Read the model definition and answer for the solid it produces. Units are mm, in the model's axes. A direction names the side the tool comes from. Give positions to 0.01 mm unless a question says otherwise; leave off trailing zeros. Write each loop counter-clockwise with the first axis right and the second up, starting at its lowest first coordinate (ties: lowest second). Pieces come first, ordered by that corner, then holes. Notation, with made-up numbers: M 60,89.25 L 107,89.25 A18 ccw 107,113.25 Z; hole C 74,15.5 d8. An arc over 180 degrees is marked long. Answer as CSV lines item,"result". Start each with the question number.
```python
from build123d import *

# Parameters (mm, degrees)
PROFILE_W                = 12.7
PROFILE_H                = 22.86
PROFILE_W_2              = 6.35
PROFILE_H_2              = 12.7
BOSS_EXTRUDE1_DEPTH      = 12.7
SKETCH7_W                = 19.05
SKETCH7_H                = 12.7
BOSS_EXTRUDE2_DEPTH      = 25.4
CUT_EXTRUDE1_DEPTH       = 37.45585824
CUT_EXTRUDE1_DEPTH_BACK  = 37.45585824
SCREWHOLE_R              = 2.159
CUT_EXTRUDE2_START       = -4.064
SKETCH3_R                = 3.683
SKETCH3_R_2              = 2.159
CUT_EXTRUDE2_DEPTH       = 4.064
BOSS_EXTRUDE4_DEPTH      = 31.75
BOSS_EXTRUDE4_DEPTH_BACK = 31.75
SKETCH11_W               = 12.7
SKETCH11_H               = 22.86
SKETCH14_R               = 2.7051
CUT_EXTRUDE3_DEPTH       = 8.89
SKETCH13_R               = 1.143
CUT_EXTRUDE4_DEPTH       = 8.89
FILLET1_R                = 6.35


with BuildPart() as part:
    # Profile → Boss-Extrude1 (new, symmetric)
    with BuildSketch(Plane.XY):
        with Locations((0, 11.43)):
            Rectangle(PROFILE_W, PROFILE_H)
        with Locations((3.175, -6.35)):
            Rectangle(PROFILE_W_2, PROFILE_H_2)
    extrude(amount=BOSS_EXTRUDE1_DEPTH, both=True)

    # Sketch7 → Boss-Extrude2 (add)
    with BuildSketch(Plane.XY.offset(12.7)):
        with Locations((-9.525, -6.35)):
            Rectangle(SKETCH7_W, SKETCH7_H)
    extrude(amount=-BOSS_EXTRUDE2_DEPTH)

    # ScrewHole → Cut-Extrude1 (cut, two sides: drawn at the far end of the back side and taken through both)
    with BuildSketch(Plane.ZY.offset(19.05).offset(-CUT_EXTRUDE1_DEPTH_BACK)):
        with Locations(Location((6.35, -6.477, 0), (0, 0, 270))):
            Circle(SCREWHOLE_R)
        with Locations(Location((-6.35, -6.477, 0), (0, 0, 270))):
            Circle(SCREWHOLE_R)
    extrude(amount=CUT_EXTRUDE1_DEPTH + CUT_EXTRUDE1_DEPTH_BACK, mode=Mode.SUBTRACT)

    # Sketch3 → Cut-Extrude2 (cut)
    # profile 1 of 2: a face of its own
    with BuildSketch(Plane(origin=(6.35, 0, 0), x_dir=(0, 0, -1), z_dir=(1, 0, 0)).offset(CUT_EXTRUDE2_START)):
        with Locations(Location((-6.35, -6.477, 0), (0, 0, 90))):
            Circle(SKETCH3_R)
        with Locations(Location((-6.35, -6.477, 0), (0, 0, 270))):
            Circle(SKETCH3_R_2, mode=Mode.SUBTRACT)
    # profile 2 of 2: a face of its own
    with BuildSketch(Plane(origin=(6.35, 0, 0), x_dir=(0, 0, -1), z_dir=(1, 0, 0)).offset(CUT_EXTRUDE2_START)):
        with Locations(Location((6.35, -6.477, 0), (0, 0, 90))):
            Circle(SKETCH3_R)
    extrude(amount=CUT_EXTRUDE2_DEPTH, mode=Mode.SUBTRACT)

    # Sketch11 → Boss-Extrude4 (add, two sides: drawn at the far end of the back side and taken through both)
    with BuildSketch(Plane.XY.offset(-BOSS_EXTRUDE4_DEPTH_BACK)):
        with Locations((0, 11.43)):
            Rectangle(SKETCH11_W, SKETCH11_H)
    extrude(amount=BOSS_EXTRUDE4_DEPTH + BOSS_EXTRUDE4_DEPTH_BACK)

    # Sketch14 → Cut-Extrude3 (cut)
    with BuildSketch(Plane(origin=(6.35, 0, 0), x_dir=(0, 0, -1), z_dir=(1, 0, 0))):
        with Locations(Location((-25.4, 11.43, 0), (0, 0, 90))):
            Circle(SKETCH14_R)
        with Locations(Location((0, 11.43, 0), (0, 0, 90))):
            Circle(SKETCH14_R)
    extrude(amount=-CUT_EXTRUDE3_DEPTH, mode=Mode.SUBTRACT)

    # Sketch13 → Cut-Extrude4 (cut)
    with BuildSketch(Plane.ZY.offset(6.35)):
        with Locations(Location((-26.67, 17.78, 0), (0, 0, 270))):
            Circle(SKETCH13_R)
        with Locations(Location((-6.35, 17.78, 0), (0, 0, 270))):
            Circle(SKETCH13_R)
        with Locations(Location((-6.35, 5.08, 0), (0, 0, 270))):
            Circle(SKETCH13_R)
        with Locations(Location((-26.67, 5.08, 0), (0, 0, 270))):
            Circle(SKETCH13_R)
    extrude(amount=-CUT_EXTRUDE4_DEPTH, mode=Mode.SUBTRACT)

    # Fillet1
    fillet1_edges = [part.edges().sort_by_distance(p)[0] for p in [
        (-6.35, -12.7, -12.7),
        (-6.35, -12.7, 12.7),
        (0, 0, 31.75),
        (0, 22.86, 31.75),
        (0, 22.86, -31.75),
        (0, 0, -31.75),
        (0, 0, -12.7),
        (0, 0, 12.7),
    ]]
    fillet(fillet1_edges, radius=FILLET1_R - 0.0001)  # a hair under: the kernel refuses the full size


solid = part.part
```
1. Given pin 1 (4.5 mm diameter, centred on y = 11.43, z = 0, fed in from -X); pin 2 (4 mm diameter, centred on x = -6, y = -4.5, fed in from -Z); pin 3 (1.8 mm diameter, centred on y = 17.78, z = -26.67, fed in from -X), each flat-ended and moving along its own axis, determine where each tip first touches the part or whether it passes through.
2. Find section B-B on z = 0. Determine the outline of the cut face in (x, y).
3. Determine the mould class of faces 1 (the face through (2.286, -7, 4)), 2 (the face through (0, 12, 31.75)), 3 (the face through (0, 22.86, 0)) for opening direction Y: +Y half, -Y half, draft (parallel to the pull), parting line (faces both ways), or undercut.
4. Find section A-A on x = -8. Determine the outline of the cut face in (y, z).
5. Find the intervals of material crossed by line 1 (Z direction, x = 3.75, y = 11.43); line 2 (Z direction, x = 0.5, y = 5.08); line 3 (X direction, y = 3.5, z = 26), in increasing order. Write a range as [from, to].
6. Find section D-D on y = -1. Determine the outline of the cut face in (x, z), then the cut area to 3 significant figures.
7. For faces 4 (the face through (-1.967, 16.724, -27.108)), 5 (the face through (0, 0, -22)), 6 (the face through (-8.23, -6.2, 8.49)), 7 (the face through (4.29, -7.275, -9.945)), determine the directions among +Z, -Z, +X, -X, +Y, -Y from which every point of the face is accessible in a straight line to the end or side of a thin tool.
8. Find section C-C on y = 11.43. Determine the outline of the cut face in (x, z).
Computed:
1,pin 1,"stops at x = -6.35"
1,pin 2,"stops at z = -14"
1,pin 3,"stops at x = 2.54"
2,outline,"M -19.05,-12.7 L 6.35,-12.7 L 6.35,8.72 L -2.54,8.72 L -2.54,14.14 L 6.35,14.14 L 6.35,22.86 L -6.35,22.86 L -6.35,0 L -19.05,0 Z"
3,face 1,"undercut"
3,face 2,"draft"
3,face 3,"+Y half"
4,outline,"M -12.7,-6.35 A6.35 ccw -6.35,-12.7 L 0,-12.7 L 0,12.7 L -6.35,12.7 A6.35 ccw -12.7,6.35 Z; hole C -6.48,-6.35 d4.32; hole C -6.48,6.35 d4.32"
5,line 1,"z = [-31.75, -2.71], [2.71, 22.69], [28.11, 31.75]"
5,line 2,"z = [-31.62, -27.81], [-25.53, -7.49], [-5.21, 31.62]"
5,line 3,"x = [-6.35, 6.35]"
6,outline,"M -19.05,-12.7 L -6.35,-12.7 L -6.35,-15.63 L 6.35,-15.63 L 6.35,15.63 L -6.35,15.63 L -6.35,12.7 L -19.05,12.7 Z"
6,area,"720 mm^2"
7,face 4,"-X"
7,face 5,"-Z, +X, -X, -Y"
7,face 6,"+X, -X"
7,face 7,"+X"
8,outline,"M -6.35,-31.75 L 6.35,-31.75 L 6.35,-2.71 L -2.54,-2.71 L -2.54,2.71 L 6.35,2.71 L 6.35,22.69 L -2.54,22.69 L -2.54,28.11 L 6.35,28.11 L 6.35,31.75 L -6.35,31.75 Z"
